Here's how the part is built. I have some questions about the finished solid (model axes, mm). Coordinates: 2 decimals unless noted, no trailing zeros. Write each loop counter-clockwise with the first axis right and the second up, starting at its lowest first coordinate (ties: lowest second). Pieces come first, ordered by that corner, then holes.
Item 1: If I drill on line 1 (X direction, y = -2.3, z = 0); line 2 (X direction, y = -3.8, z = 0); line 3 (Z direction, x = 5, y = -3), over which ranges is the centre line in solid material (lowest first)?
Item 2: We'd pull the mould along Z, two halves only. Please class faces 1 (the face through (-7.73, -5.09, -24.55)), 2 (the face through (-1.231, -4.22, 27.973)), 3 (the face through (18.5, -8, -18.5)), 4 (the face through (-9.49, -0.26, -22.89)): +Z half, -Z half, draft (parallel to the pull), parting line (faces both ways), or undercut.
Item 3: I'm going to push flat-ended pins straight in: pin 1 Ø1 at (x, y) = (9, -5) entering from -Z; pin 2 Ø1.5 at (x, z) = (-20, 20) entering from -Y. Where does each tip first touch, or does it pass through?
Item 4: If we section it at A-A (y = -3.75): Please give me the cut outline in (x, z), then the cut area to 3 significant figures.
from build123d import *

# Parameters (mm, degrees)
SKETCH_1_R               = 28
EXTRUDE_1_DEPTH          = 2
SKETCH_4_R               = 23.5
CUT_EXTRUDE_1_DEPTH      = 41.841155713
CUT_EXTRUDE_START        = -0.6
SKETCH_5_R               = 28
CUT_EXTRUDE_2_DEPTH      = 0.6
CHAMFER_1_SIZE           = 1.2
CHAMFER_2_SIZE           = 1.732
CHAMFER_2_SIZE2          = 0.999970666
CUT_REVOLVE_1_ANGLE      = 45
PATTERN_CIRCULAR_1_COUNT = 4
SKETCH_8_R               = 24.78
SKETCH_8_R_2             = 24.32
EXTRUDE_2_DEPTH          = 0.5


with BuildPart() as part:
    # 草图1 → 凸台-拉伸1 (new body)
    with BuildSketch(Plane(origin=(0, 0, 0), x_dir=(1, 0, 0), z_dir=(0, 1, 0))):
        with Locations(Location((0, 0, 0), (0, 0, 270))):
            Circle(SKETCH_1_R)
    extrude(amount=EXTRUDE_1_DEPTH)

    # 草图2 → 旋转1 (revolve)
    with BuildSketch(Plane(origin=(0, 0, 0), x_dir=(-0.9702957262759954, 0, -0.24192189559967248), z_dir=(0.24192189559967245, 0, -0.9702957262759953)), mode=Mode.PRIVATE) as revolve_1_sk:
        with BuildLine():
            Line((25.93, -8), (25.93, -7.5))
            Line((25.93, -7.5), (25.505, -7.075))
            Line((25.505, -7.075), (25.93, -6.65))
            Line((25.93, -6.65), (25.93, -5.8))
            Line((25.93, -5.8), (25.74, -5.61))
            Line((25.74, -5.61), (25.74, -4.59))
            Line((25.74, -4.59), (25.93, -4.4))
            Line((25.93, -4.4), (25.93, -3))
            Line((25.93, -3), (25.74, -2.81))
            Line((25.74, -2.81), (25.74, -1.79))
            Line((25.74, -1.79), (25.93, -1.6))
            Line((25.93, -1.6), (25.93, -1.4))
            ThreePointArc((25.93, -1.4), (25.519949494, -0.410050506), (24.53, 0))
            Line((24.53, 0), (28, 0))
            Line((28, 0), (28, -8))
            Line((28, -8), (25.93, -8))
        make_face()
    revolve(revolve_1_sk.sketch.rotate(Axis((0, 0, 0), (0, 1, 0)), 284), axis=Axis((0, 0, 0), (0, 1, 0)))

    # 草图4 → 切除-拉伸1 (cut, through all)
    with BuildSketch(Plane(origin=(0, 2, 0), x_dir=(1, 0, 0), z_dir=(0, 1, 0))):
        with Locations(Location((0, 0, 0), (0, 0, 270))):
            Circle(SKETCH_4_R)
    extrude(amount=-CUT_EXTRUDE_1_DEPTH, mode=Mode.SUBTRACT)

    # 草图5 → 切除-拉伸2 (cut)
    with BuildSketch(Plane(origin=(0, 2, 0), x_dir=(1, 0, 0), z_dir=(0, 1, 0)).offset(CUT_EXTRUDE_START)):
        with Locations(Location((0, 0, 0), (0, 0, 90))):
            Circle(SKETCH_5_R)
    extrude(amount=CUT_EXTRUDE_2_DEPTH, mode=Mode.SUBTRACT)

    # 倒角1
    chamfer_1_edges = [part.edges().sort_by_distance(p)[0] for p in [
        (0, 1.4, -23.5),
    ]]
    chamfer(chamfer_1_edges, length=CHAMFER_1_SIZE)

    # 倒角2
    chamfer_2_edges = [part.edges().sort_by_distance(p)[0] for p in [
        (0, 1.4, -28),
    ]]
    chamfer_2_side = [part.faces().sort_by_distance(p)[0] for p in [
        (0, 0.7, -28),
    ]]
    chamfer(chamfer_2_edges, length=CHAMFER_2_SIZE, length2=CHAMFER_2_SIZE2, reference=chamfer_2_side[0])

    # 草图7 → 切除-旋转1 (revolve, cut)
    with BuildSketch(Plane.XY):
        Polygon((28, -8), (28, -7), (27, -8), align=None)
    cut_revolve_1 = revolve(axis=Axis((0, 0, 0), (0, 1, 0)), revolution_arc=CUT_REVOLVE_1_ANGLE, mode=Mode.SUBTRACT)

    # 阵列(圆周)1: 切除-旋转1 ×4 about axis
    pattern_circular_1_axis = Axis((0, 0, 0), (0, 1, 0))
    for i in range(1, PATTERN_CIRCULAR_1_COUNT):
        add(cut_revolve_1.rotate(pattern_circular_1_axis, i * 360 / PATTERN_CIRCULAR_1_COUNT), mode=Mode.SUBTRACT)

    # 草图8 → 凸台-拉伸2 (add)
    with BuildSketch(Plane.XZ):
        with Locations(Location((0, 0, 0), (0, 0, 270))):
            Circle(SKETCH_8_R)
        with Locations(Location((0, 0, 0), (0, 0, 270))):
            Circle(SKETCH_8_R_2, mode=Mode.SUBTRACT)
    extrude(amount=EXTRUDE_2_DEPTH)


solid = part.part
Answer list:
1. line 1: x = -28 to -25.74, 25.74 to 28
1. line 2: x = -28 to -25.93, 25.93 to 28
1. line 3: z = -27.55 to -25.44, 25.44 to 27.55
2. face 1: undercut
2. face 2: parting line
2. face 3: draft
2. face 4: undercut
3. pin 1: stops at z = -26.68
3. pin 2: stops at y = -8
4. outline: circle Ø56 at (0, 0); hole circle Ø51.86 at (0, 0)
4. area: 351 mm2
